Input: part model. Units: mm. Frame: model coordinates. A direction names the side the tool comes from. Give positions to 0.01 mm unless a question says otherwise; leave off trailing zeros. Loops run counter-clockwise (first coordinate to the right, second up) from the corner with the lowest first, then second, coordinate; pieces in that order, holes last. Notation, with made-up numbers: M 22.25,-5 L 38.25,-5 A30 ccw 38.25,19 Z; hole C -12,26.25 d6. An arc over 180 degrees is marked long. Return JSON: item names as keys, results as strings. Group by question number.
```python
from build123d import *

# Parameters (mm, degrees)
F1_DEPTH = 25.4
F2_W     = 151.775382
F2_H     = 131.256286
F3_DEPTH = 25.4
F4_R     = 6.35
F5_DEPTH = 15.24


with BuildPart() as f1:
    # F0 (on Front) → F1 (new body)
    with BuildSketch(Plane.XZ):
        Polygon((-75.533889, 76.327696), (-75.533889, 61.938155), (-75.533889, -75.790301), (72.815411, -75.790301), (76.241493, -75.790301), (76.241493, 76.327696), align=None)
    extrude(amount=F1_DEPTH)

    # F2 (on face) → F3 (join)
    with BuildSketch(Plane(origin=(0, 0, 0), x_dir=(-1, 0, 0), z_dir=(0, 1, 0))):
        with Locations((-0.353802, -10.162158)):
            Rectangle(F2_W, F2_H)
    extrude(amount=F3_DEPTH)

    # F4 (on face) → F5 (cut)
    with BuildSketch(Plane(origin=(0, 0, 0), x_dir=(-1, 0, 0), z_dir=(0, 1, 0))):
        with Locations((-55.87405, 65.896841)):
            Circle(F4_R)
        with Locations((0, 65.896851)):
            Circle(F4_R)
        with Locations((51.929399, 65.896851)):
            Circle(F4_R)
    extrude(amount=-F5_DEPTH, mode=Mode.SUBTRACT)


solid = f1.part
```
Item 1: Section D-D, the plane x = 25. Return loops of the section in (y, z).
Item 2: Section C-C, the plane z = 63. Return loops of the section in (x, y).
Item 3: Material intervals for line 1 (Z direction, x = 0, y = -7.75); line 2 (Z direction, x = 62, y = 11.5), sorted ascending. Write a range as from..to.
Item 4: Reachability of faces 5 (the face through (-1, 0, 59)), 6 (the face through (1, -13, 76.328)), 7 (the face through (-55.343, -7.513, 71.251)) from +Z, -Z, +X, -X, +Y, -Y: full face, straight path, thin tool, end or side. Return the list, or none.
Item 5: Section A-A, the plane x = 0. Return loops of the section in (y, z).
Item 6: Pull-direction query (Z, two-part tool) for faces 1 (the face through (1, 0, -75.79)), 2 (the face through (56, -15.24, 66)), 3 (the face through (57.251, -7.513, 59.698)), 4 (the face through (-75.534, 0, -1)); classes: pulls with the +Z half, pulls with the -Z half, needs draft (parallel to the pull), parting line crosses it, or undercut.
Item 7: First-contact query: pin 1 Ø4 at (x, z) = (-49.5, 66.5) entering from +Y; pin 2 Ø6.5 at (x, z) = (-7, 64.5) entering from +Y; pin 3 Ø12.5 at (x, y) = (10.5, 13) entering from +Z. Flat tips, straight axial feed; report the tip coordinate or a pass-through.
Item 8: Section B-B, the plane y = 7. Return loops of the section in (x, z), then the cut area to 3 significant figures.
Answer below:
{
 "1": {"outline": "M -25.4,-75.79 L 25.4,-75.79 L 25.4,55.47 L 0,55.47 L 0,76.33 L -25.4,76.33 Z"},
 "2": {"outline": "M -75.53,-25.4 L 76.24,-25.4 L 76.24,0 L 61.52,0 L 61.52,-15.24 L 50.22,-15.24 L 50.22,0 L 5.65,0 L 5.65,-15.24 L -5.65,-15.24 L -5.65,0 L -46.28,0 L -46.28,-15.24 L -57.58,-15.24 L -57.58,0 L -75.53,0 Z"},
 "3": {"line 1": "-75.79..59.55, 72.25..76.33", "line 2": "-75.79..55.47"},
 "4": {"face 5": "+Z, +X, -X, +Y", "face 6": "+Z, +X, -X, +Y, -Y", "face 7": "+Y"},
 "5": {"outline": "M -25.4,-75.79 L 25.4,-75.79 L 25.4,55.47 L 0,55.47 L 0,59.55 L -15.24,59.55 L -15.24,72.25 L 0,72.25 L 0,76.33 L -25.4,76.33 Z"},
 "6": {"face 1": "pulls with the -Z half", "face 2": "undercut", "face 3": "undercut", "face 4": "needs draft"},
 "7": {"pin 1": "y = -15.24", "pin 2": "y = 0", "pin 3": "z = 55.47"},
 "8": {"outline": "M -75.53,-75.79 L 76.24,-75.79 L 76.24,55.47 L -75.53,55.47 Z", "area": "19,900 mm^2"}
}
